from build123d import *

# Parameters (mm, degrees)
IZIM1_W                     = 104
IZIM1_H                     = 50
Y_KSEKLIK_EKSTR_ZYON1_DEPTH = 3


with BuildPart() as part:
    # Çizim1 → Yükseklik-Ekstrüzyon1 (new body)
    with BuildSketch(Plane(origin=(0, 0, 0), x_dir=(1, 0, 0), z_dir=(0, 1, 0))):
        with Locations((52, -25)):
            Rectangle(IZIM1_W, IZIM1_H)
        with BuildLine():
            Line((42.5, -10), (61.5, -10))
            ThreePointArc((61.5, -10), (63.621320344, -10.878679656), (64.5, -13))
            Line((64.5, -13), (64.5, -22))
            ThreePointArc((64.5, -22), (63.621320344, -24.121320344), (61.5, -25))
            Line((61.5, -25), (42.5, -25))
            ThreePointArc((42.5, -25), (40.378679656, -24.121320344), (39.5, -22))
            Line((39.5, -22), (39.5, -13))
            ThreePointArc((39.5, -13), (40.378679656, -10.878679656), (42.5, -10))
        make_face(mode=Mode.SUBTRACT)
    extrude(amount=Y_KSEKLIK_EKSTR_ZYON1_DEPTH)


solid = part.part
Could you check a few things on this model? Use its own coordinates, in mm. A direction names the side the tool comes from. Give positions to 0.01 mm unless a question says otherwise; leave off trailing zeros. Order: outer loops, then holes, each group sorted by start corner. A loop starts at its lowest first (then second) coordinate and runs counter-clockwise, first axis right, second up.
Item 1: If we mould it in two halves opening along Z, with no side actions, what happens to faces 3 (the face through (52, 1, 10)), 4 (the face through (51, 3, 30)), 5 (the face through (39.5, 1, 18)), 6 (the face through (51, 1, 50))? For each: pulls with the +Z half, pulls with the -Z half, needs draft (parallel to the pull), parting line crosses it, or undercut.
Item 2: If we section it at A-A, the plane z = 16.5: Write out the boundary of the cut face in (x, y), plus the area to 3 significant figures.
Item 3: If we section it at B-B, the plane y = 0.9: Write out the boundary of the cut face in (x, z), plus the area to 3 significant figures.
Item 4: I need wall thicknesses on line 1 (X direction, y = 1.8, z = 22); line 2 (Z direction, x = 58.5, y = 0.75); line 3 (Z direction, x = 62.5, y = 1.6). Which ranges of each line are inside material? Lowest first, please.
Item 5: If we section it at C-C, the plane x = 63.5: Write out the boundary of the cut face in (y, z), plus the area to 3 significant figures.
Item 6: For faces 1 (the face through (104, 1, 25)), 2 (the face through (63.64, 1.48, 24.1)), which set-ups out of +Z, -Z, +X, -X, +Y, -Y let a thin tool reach every point of the face, with its end or its side?
Values:
1. face 3: undercut
1. face 4: needs draft
1. face 5: undercut
1. face 6: pulls with the +Z half
2. outline: (0, 0) - (39.5, 0) - (39.5, 3) - (0, 3) - close; (64.5, 0) - (104, 0) - (104, 3) - (64.5, 3) - close
2. area: 237 mm2
3. outline: (0, 0) - (104, 0) - (104, 50) - (0, 50) - close; hole (39.5, 13) arc R3 ccw to (42.5, 10) - (61.5, 10) arc R3 ccw to (64.5, 13) - (64.5, 22) arc R3 ccw to (61.5, 25) - (42.5, 25) arc R3 ccw to (39.5, 22) - close
3. area: 4,830 mm2
4. line 1: x = 0 to 39.5, 64.5 to 104
4. line 2: z = 0 to 10, 25 to 50
4. line 3: z = 0 to 10.17, 24.83 to 50
5. outline: (0, 0) - (3, 0) - (3, 10.76) - (0, 10.76) - close; (0, 24.24) - (3, 24.24) - (3, 50) - (0, 50) - close
5. area: 110 mm2
6. face 1: +Z, -Z, +X, +Y, -Y
6. face 2: +Y, -Y
